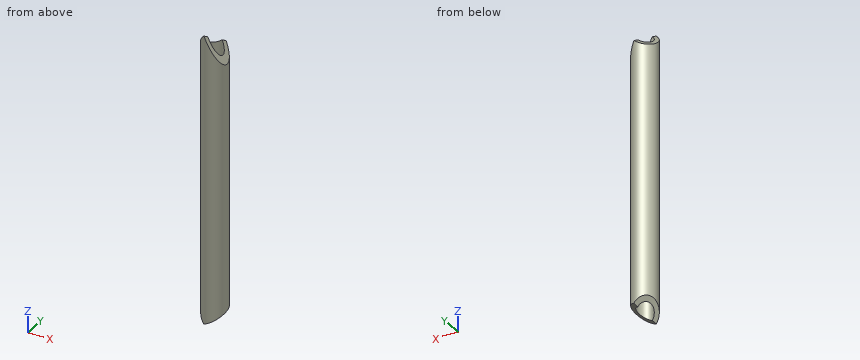
Autodesk Inventor part; units mm, degrees
ref_plane "Start Plane" through (0, 0, -4.9897) normal (0, 0, 1) x (1, 0, 0)
ref_plane "End Plane" through (0, 0, 247.019) normal (0, 0, 1) x (1, 0, 0)
ref_plane "Work Plane4" through (6.5371, -8.4304, 252.5558) normal (-0.4523, 0.5834, 0.6746) x (0.8778, 0.1576, 0.4523)
ref_plane "Start Plane" through (0, 0, -4.9897) normal (0, 0, 1) x (1, 0, 0)
ref_plane "End Plane" through (0, 0, 247.019) normal (0, 0, 1) x (1, 0, 0)
sketch "Sketch" plane through (0, 0, 0) normal (0, 0, 1) x (1, 0, 0)
  circle A0 centre (0, 0) radius 6.9342
  circle A1 centre (0, 0) radius 10.668
  dimension "d0" = 21.336
  dimension "d1" = 3.7338
extrude "Body" add sketch "Sketch" along normal up to surface (252.0086 mm away) from surface at -4.9897
sketch "Sketch3" plane through (0, 0, 0) normal (0, 0, 1) x (1, 0, 0)
  line L0 (0, 0) -> (10, 0)
ref_plane "Work Plane3" through (0, 0, 0) normal (0, -1, 0) x (1, 0, 0)
sketch "Sketch4" plane through (0, 0, 0) normal (0, -1, 0) x (1, 0, 0)
  line L0 (-2, -4.9897) -> (12, -4.9897)
  line L1 (-2, 247.019) -> (12, 247.019)
  dimension "d7" = 252.0086
ref_plane "Work Plane4" through (6.5371, -8.4304, 252.5558) normal (-0.4523, 0.5834, 0.6746) x (0.8778, 0.1576, 0.4523)
split "Split1" plane through (6.5371, -8.4304, 252.5558) removes the side toward (-0.4523, 0.5834, 0.6746)
ref_plane "Work Plane5" through (-10.6626, 0.3395, 260.0533) normal (0.8734, -0.0278, 0.4862) x (0.4868, 0.0163, -0.8734)
split "Split2" plane through (-10.6626, 0.3395, 260.0533) removes the side toward (0.8734, -0.0278, 0.4862)
ref_plane "Work Plane6" through (-7.2827, -7.7955, 247.658) normal (0.366, 0.3918, 0.8441) x (0.9274, -0.0778, -0.366)
split "Split3" plane through (-7.2827, -7.7955, 247.658) removes the side toward (0.366, 0.3918, 0.8441)
ref_plane "Work Plane7" through (6.5371, -8.4304, -9.7489) normal (-0.4134, 0.5331, -0.7382) x (0.3473, 0.8417, 0.4134)
split "Split4" plane through (6.5371, -8.4304, -9.7489) removes the side toward (-0.4134, 0.5331, -0.7382)
ref_plane "Work Plane8" through (-9.643, -4.5628, -6.8509) normal (0.4884, 0.2311, -0.8414) x (-0.5046, -0.7119, -0.4884)
split "Split5" plane through (-9.643, -4.5628, -6.8509) removes the side toward (0.4884, 0.2311, -0.8414)
equation "\"d0\" = G_H"
equation "\"d1\" = G_T"
equation "\"d2\" = G_L"
equation "\"G_H\" = 21.336"
equation "\"G_T\" = 3.7338"
equation "\"G_L\" = 252.00865"
equation "\"G_OFFSET_START\" = 4.98966"
equation "\"G_OFFSET_END\" = 6.13701"
equation "\"d4\" = -G_OFFSET_START"
equation "\"d5\" = G_OFFSET_END + B_L"
equation "\"B_L\" = 240.88198"
properties part number "ANSI - 1/2 x 0.147 - 9.922" material "Steel, Mild"
For this review, take the finished solid that the model builds, in its own axes (mm). Round coordinates to 2 decimals unless told otherwise and drop trailing zeros. Write each loop counter-clockwise with the first axis right and the second up, starting at its lowest first coordinate (ties: lowest second). Pieces come first, ordered by that corner, then holes. Notation, with made-up numbers: M 57,60.25 L 70,60.25 A21 cw 70,81.25 Z; hole C 73.25,65 d8. An arc over 180 degrees is marked long. Write item = value, one per line. Start each with the question number.
(1) Clearance check with flat-ended pins moving along their axes: pin 1 Ø8 at (x, y) = (4, 2.5) entering from -Z; pin 2 Ø3 at (x, y) = (1.5, -8) entering from +Z; pin 3 Ø6 at (y, z) = (-8, 62) entering from -X. State where each tip first meets the part, or that it passes through.
(2) For line 1 along Y through (x, z) = (0, 53.5); line 2 along Y through (x, z) = (-5.75, 216), list the stretches that pass through material, from the lowest coordinate up.
(3) We need section B-B (x = 0). Give the boundary of the cut face in (y, z), then the cut area to 3 significant figures.
(4) We need section C-C (z = 182). Give the boundary of the cut face in (x, y).
(5) We need section A-A (y = 0). Give the boundary of the cut face in (x, z).
Results found:
q1.pin_1 = 3.38
q1.pin_2 = 240.42
q1.pin_3 = -9.42
q2.line_1 = -10.67 to -6.93, 6.93 to 10.67
q2.line_2 = -8.99 to -3.88, 3.88 to 8.99
q3.outline = M -10.67,-2.93 L -6.93,-1.9 L -6.93,240.48 L -10.67,240.27 Z; M 6.93,5.01 L 10.67,7.7 L 10.67,231.66 L 6.93,234.89 Z
q3.area = 1,750 mm²
q4.outline = C 0,0 d21.34; hole C 0,0 d13.87
q5.outline = M -10.67,5.97 L -6.93,3.88 L -6.93,236.23 L -10.67,233.73 Z; M 6.93,4.02 L 10.67,6.19 L 10.67,221.72 L 6.93,228.42 Z
